For this review, take the finished solid that the model builds, in its own axes (mm). Face numbers are marked on the shaded views. Round coordinates to 2 decimals unless told otherwise and drop trailing zeros. Write each loop counter-clockwise with the first axis right and the second up, starting at its lowest first coordinate (ties: lowest second). Pieces come first, ordered by that corner, then holes.
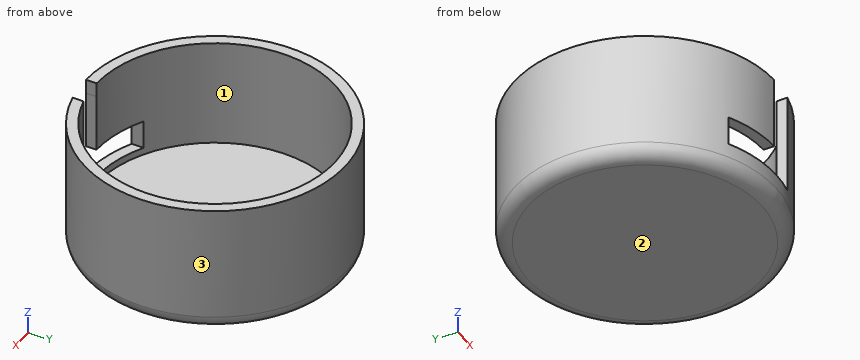
from build123d import *

# Parameters (mm, degrees)
F0_R     = 18.2
F0_R_2   = 16.7
F1_DEPTH = 3
F2_R     = 18.2
F2_R_2   = 16.7
F3_DEPTH = 15
F6_DEPTH = 10
F7_R     = 2


with BuildPart() as f1:
    # F0 (on Top) → F1 (new body)
    with BuildSketch(Plane.XY):
        Circle(F0_R)
        Circle(F0_R_2, mode=Mode.SUBTRACT)
        Circle(F0_R_2)
    extrude(amount=F1_DEPTH)

    # F2 (on face) → F3 (join)
    with BuildSketch(Plane.XY.offset(3)):
        Circle(F2_R)
        Circle(F2_R_2, mode=Mode.SUBTRACT)
    extrude(amount=F3_DEPTH)

    # F5 (on offset) → F6 (cut)
    with BuildSketch(Plane.XZ.offset(18.2)):
        Polygon((-0.037793, 15.999911), (0, 8), (-8, 8), (-8, 4), (4, 4), (4, 20), (3.962207, 19.999911), (-0.037793, 19.999911), align=None)
    extrude(amount=-F6_DEPTH, mode=Mode.SUBTRACT)

    # F7
    f7_edges = [f1.edges().sort_by_distance(p)[0] for p in [
        (-18.2, 0, 0),
    ]]
    fillet(f7_edges, radius=F7_R)


solid = f1.part
(1) We need section D-D, the plane z = 11.75. Give the boundary of the cut face in (x, y) (3 decimals), and give its area (3 significant figures).
Geometry check:
outline: (-0.018, -18.2) - (-0.018, -16.7) arc R16.7 cw (long way) to (4, -16.214) - (4, -17.755) arc R18.2 ccw (long way) to start
area: 158 mm2
(2) We need section B-B, the plane z = 3.5. Give the boundary of the cut face in (x, y).
Geometry check:
outline: circle Ø36.4 at (0, 0); hole circle Ø33.4 at (0, 0)
(3) Mouldability with a two-part tool opening along Y and no side actions: class the marked faces 1, 2 and 3 as pulls with the +Y half, pulls with the -Y half, needs draft (parallel to the pull), parting line crosses it, or undercut.
Geometry check:
face 1: undercut
face 2: needs draft
face 3: parting line crosses it
(4) We need section C-C, the plane z = 6.75. Give the boundary of the cut face in (x, y) (3 decimals).
Geometry check:
outline: (-8, -16.347) - (-8, -14.659) arc R16.7 cw (long way) to (4, -16.214) - (4, -17.755) arc R18.2 ccw (long way) to start
(5) We need section A-A, the plane y = 0. Give the boundary of the cut face in (x, z).
Geometry check:
outline: (-18.2, 2) arc R2 ccw to (-16.2, 0) - (16.2, 0) arc R2 ccw to (18.2, 2) - (18.2, 18) - (16.7, 18) - (16.7, 3) - (-16.7, 3) - (-16.7, 18) - (-18.2, 18) - close
(6) For line 1 along X through (y, z) = (0, 8.75); line 2 along Z through (x, y) = (-11, 10); line 3 along Y through (x, z) = (0.5, 17.25), list the stretches that pass through material, from the lowest coordinate up.
Geometry check:
line 1: x = -18.2 to -16.7, 16.7 to 18.2
line 2: z = 0 to 3
line 3: y = 16.69 to 18.19
(7) For pin 1 Ø8 at (x, y) = (5.5, 8.5) entering from +Z; pin 2 Ø1.5 at (y, z) = (-13.5, 3) entering from +X; pin 3 Ø1.8 at (x, y) = (-2, -16) entering from +Z; pin 4 Ø0.8 at (y, z) = (-15.5, 6.5) entering from +X, all flat-tipped, find the tip position at first contact; note any pin that passes through.
Geometry check:
pin 1: stops at z = 3
pin 2: stops at x = 12.99
pin 3: stops at z = 18
pin 4: stops at x = 10.16
